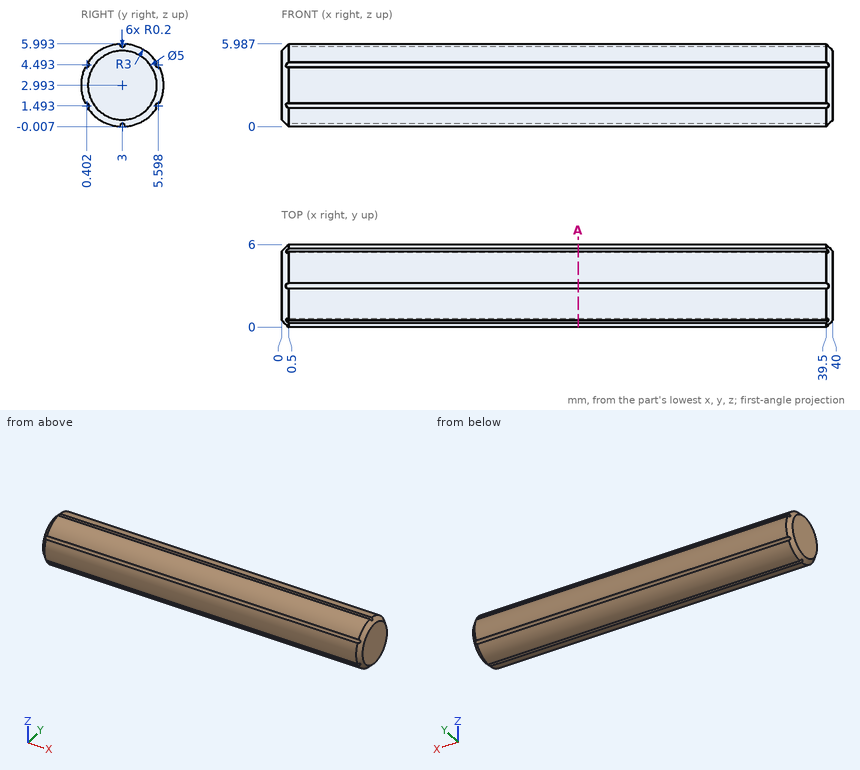
Print and shaded views of the part. All mm, measured from the part's lowest x, y and z. Give positions to 0.01 mm unless a question says otherwise; leave off trailing zeros. Write each loop counter-clockwise with the first axis right and the second up, starting at its lowest first coordinate (ties: lowest second). Pieces come first, ordered by that corner, then holes. Notation, with made-up numbers: (40, 48) -> (83, 48) arc R17 ccw to (83, 65) -> close; hole circle Ø4 at (-8.5, -37). An arc over 180 degrees is marked (long way). Use CSV: the item, a comma, the result in double quotes. Start each with the question number.
1) Cut at A-A on x = 21.5. List the corners of the cut face in (y, z).
2) Pin check, flat tips, straight feed: P1, Ø2, axis at x = 4.5, y = 5, coming from the +Z side; P2, Ø1.5, axis at x = 14, y = 1.5, coming from the -Z side; P3, Ø1, axis at x = 29, y = 4.5, coming from the -Z side (1 decimal). Stop position of each tip, or through.
3) Drill centre lines: L1, parallel to Z at x = 32.5, y = 3; L2, parallel to Z at x = 32.5, y = 2.75; L3, parallel to Y at x = 21.5, z = 0.5. Where is each one in solid material? Low to high.
Final values:
1,outline,"(0.31, 1.67) arc R0.2 cw to (0.51, 1.32) arc R3 ccw to (2.8, 0) arc R0.2 cw to (3.2, 0) arc R3 ccw to (5.49, 1.32) arc R0.2 cw to (5.69, 1.67) arc R3 ccw to (5.69, 4.32) arc R0.2 cw to (5.49, 4.66) arc R3 ccw to (3.2, 5.99) arc R0.2 cw to (2.8, 5.99) arc R3 ccw to (0.51, 4.66) arc R0.2 cw to (0.31, 4.32) arc R3 ccw to start"
2,P1,"stops at z = 5.82"
2,P2,"stops at z = 0.09"
2,P3,"stops at z = 0.2"
3,L1,"z = 0.19 to 5.79"
3,L2,"z = 0 to 5.98"
3,L3,"y = 1.33 to 4.67"
